Input: dimensioned drawing with shaded views. Units: mm. Origin: part minimum x, y, z. Round coordinates to 2 decimals unless told otherwise and drop trailing zeros. Order: outer loops, then holes, each group sorted by start corner. A loop starts at its lowest first (then second) coordinate and runs counter-clockwise, first axis right, second up. Notation, with made-up numbers: (-12, -26) - (-6, -26) arc R8 cw to (-6, -17) - close; hole circle Ø8 at (18.5, 82). An arc over 180 degrees is marked (long way). Return JSON: item names as keys, results as strings. Group by question number.
1) Section D-D, the plane x = 7.75. Return loops of the section in (y, z).
2) Contact query for flat-ended pins moving along their axis: P1, Ø2, axis at x = 16.5, y = 3.5, coming from the -Z side; P2, Ø6, axis at x = 13.5, z = 10, coming from the -Y side; P3, Ø4, axis at x = 15.63, z = 6.75, coming from the +Y side; P4, Ø3, axis at y = 3, z = 13, coming from the +X side. Output: stop coordinate, or through.
3) Ray query, line 1 (Z direction, x = 8.75, y = 1) (1 decimal); line 2 (Z direction, x = 10, y = 0.9); line 3 (Y direction, x = 7.25, z = 5.75). Return the intervals inside material, ascending. Write a range as from..to.
4) Section C-C, the plane z = 6.75. Return loops of the section in (x, y), plus the area to 3 significant figures.
5) Section B-B, the plane x = 10. Return loops of the section in (y, z).
6) Section A-A, the plane z = 10. Return loops of the section in (x, y).
7) Mould query, pull axis Z, two halves, no side actions, for the marked faces 1, 2 and 3. Classes: pulls with the +Z half, pulls with the -Z half, needs draft (parallel to the pull), parting line crosses it, or undercut.
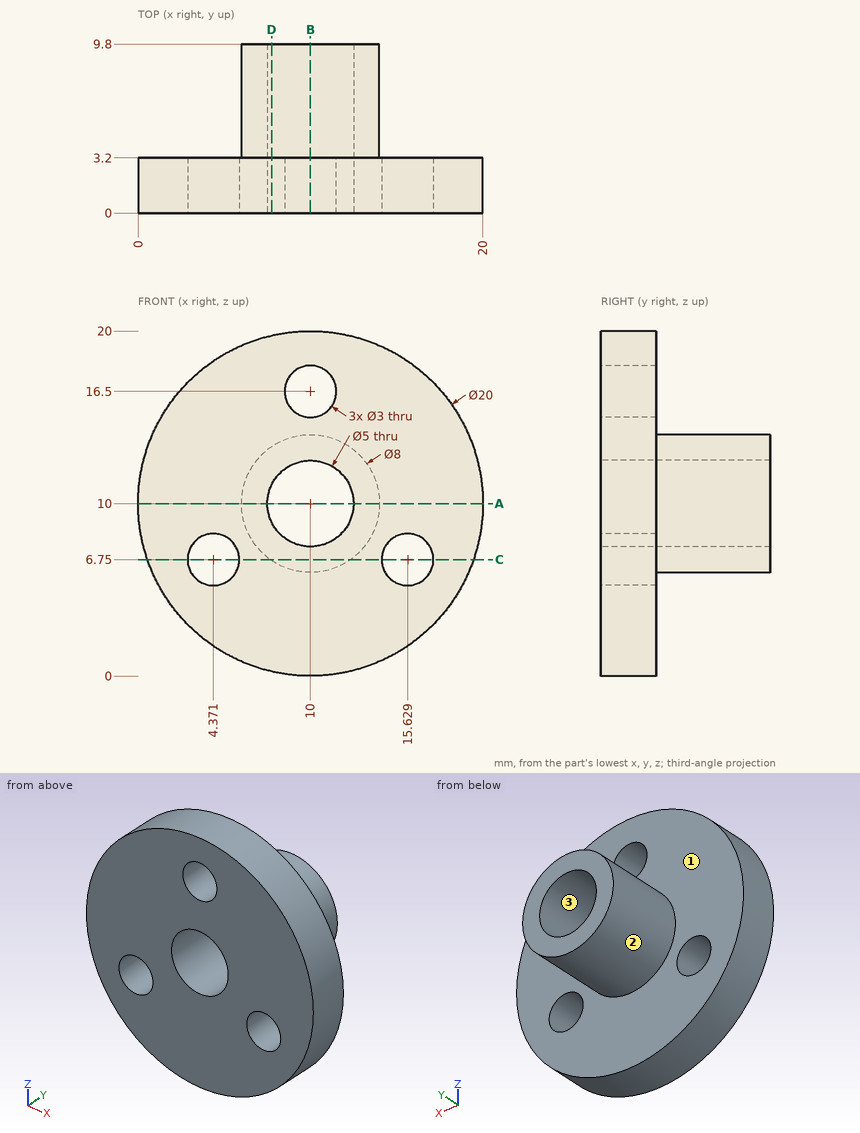
Geometry check:
{
 "1": {"outline": "(0, 0.26) - (3.2, 0.26) - (3.2, 6.69) - (9.8, 6.69) - (9.8, 8.91) - (0, 8.91) - close; (0, 11.09) - (9.8, 11.09) - (9.8, 13.31) - (3.2, 13.31) - (3.2, 19.74) - (0, 19.74) - close"},
 "2": {"P1": "z = 1.68", "P2": "y = 0", "P3": "y = 3.2", "P4": "x = 19.89"},
 "3": {"line 1": "0.1..7.8, 12.2..15.7, 17.3..19.9", "line 2": "0..7.5, 12.5..15, 18..20", "line 3": "0..3.2"},
 "4": {"outline": "(0.54, 0) - (2.87, 0) - (2.87, 3.2) - (0.54, 3.2) - close; (5.87, 0) - (14.13, 0) - (14.13, 3.2) - (12.33, 3.2) - (12.33, 9.8) - (7.67, 9.8) - (7.67, 3.2) - (5.87, 3.2) - close; (17.13, 0) - (19.46, 0) - (19.46, 3.2) - (17.13, 3.2) - close", "area": "72.1 mm2"},
 "5": {"outline": "(0, 0) - (3.2, 0) - (3.2, 6) - (9.8, 6) - (9.8, 7.5) - (0, 7.5) - close; (0, 12.5) - (9.8, 12.5) - (9.8, 14) - (3.2, 14) - (3.2, 15) - (0, 15) - close; (0, 18) - (3.2, 18) - (3.2, 20) - (0, 20) - close"},
 "6": {"outline": "(0, 0) - (7.5, 0) - (7.5, 9.8) - (6, 9.8) - (6, 3.2) - (0, 3.2) - close; (12.5, 0) - (20, 0) - (20, 3.2) - (14, 3.2) - (14, 9.8) - (12.5, 9.8) - close"},
 "7": {"face 1": "needs draft", "face 2": "parting line crosses it", "face 3": "undercut"}
}
